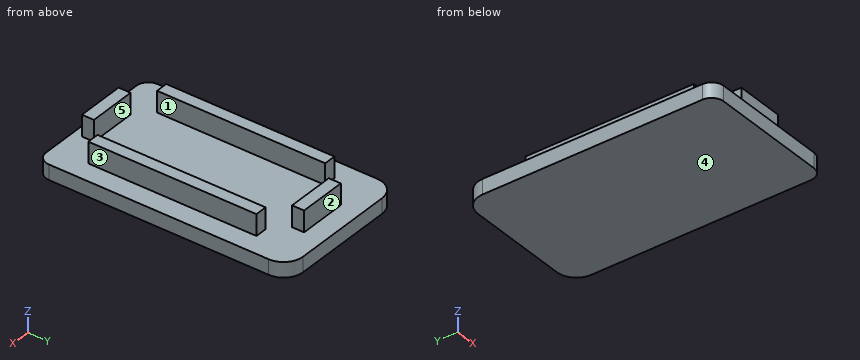
Autodesk Inventor part; units mm, degrees
ref_plane "YZ Plane" through (0, 0, 0) normal (1, 0, 0) x (0, 1, 0)
ref_plane "XZ Plane" through (0, 0, 0) normal (0, 1, 0) x (-1, 0, 0)
ref_plane "XY Plane" through (0, 0, 0) normal (0, 0, 1) x (1, 0, 0)
sketch "Boceto1" plane through (0, 0, 0) normal (0, 0, 1) x (1, 0, 0)
  line L0 (20, -40) -> (-20, -40)
  line L1 (-20, -40) -> (-20, 40)
  line L2 (-20, 40) -> (20, 40)
  line L3 (20, 40) -> (20, -40)
  line L4 (20, -40) -> (-20, 40) construction
  line L5 (-20, -40) -> (20, 40) construction
  line L6 (23.7, -43.7) -> (-23.7, -43.7)
  line L7 (-23.7, -43.7) -> (-23.7, 43.7)
  line L8 (-23.7, 43.7) -> (23.7, 43.7)
  line L9 (23.7, 43.7) -> (23.7, -43.7)
  line L10 (-23.7, -40) -> (23.7, -40)
  point P0 (0, 0)
  dimension "d0" = 40
  dimension "d1" = 80
  dimension "d2" = 3.7
  dimension "d20" = 3.7
extrude "Extrusión1" add sketch "Boceto1" along normal blind 5 contours L0 L1 L2 L3 | L3 L2 L1 L10 L7 L8 L9
sketch "Boceto2" plane through (0, 0, 5) normal (0, 0, 1) x (1, 0, 0)
  line L0 (17.5, -37.5) -> (-17.5, -37.5)
  line L1 (-17.5, -37.5) -> (-17.5, 37.5)
  line L2 (-17.5, 37.5) -> (17.5, 37.5)
  line L3 (17.5, 37.5) -> (17.5, -37.5)
  line L4 (17.5, -37.5) -> (-17.5, 37.5) construction
  line L5 (-17.5, -37.5) -> (17.5, 37.5) construction
  line L6 (17, 37) -> (-17, 37)
  line L7 (-17, 37) -> (-17, -37)
  line L8 (-17, -37) -> (17, -37)
  line L9 (17, -37) -> (17, 37)
  line L10 (-13, 33) -> (13, 33)
  line L11 (13, 33) -> (13, -33)
  line L12 (13, -33) -> (-13, -33)
  line L13 (-13, -33) -> (-13, 33)
  line L14 (8, 33) -> (8, 37)
  line L15 (-8, 33) -> (-8, 37)
  line L16 (13, 28) -> (17, 28)
  line L17 (13, -28) -> (17, -28)
  line L18 (-13, -28) -> (-17, -28)
  line L19 (-8, -33) -> (-8, -37)
  line L20 (8, -33) -> (8, -37)
  line L21 (-17, 28) -> (-13, 28)
  point P0 (0, 0)
  dimension "d5" = 35
  dimension "d6" = 75
  dimension "d7" = 0.5
  dimension "d8" = 4
  dimension "d9" = 5
  dimension "d10" = 5
  dimension "d11" = 5
  dimension "d12" = 5
  dimension "d13" = 5
  dimension "d14" = 5
  dimension "d15" = 5
  dimension "d16" = 5
extrude "Extrusión2" add sketch "Boceto2" along normal blind 7 contours L14 L10 L15 L6 | L9 L17 L11 L16 | L21 L13 L18 L7 | L8 L19 L12 L20
fillet "Empalme1" radius 6.5 2 edges at (23.7, 43.7, 2.5) (-23.7, 43.7, 2.5)
fillet "Empalme2" radius 4 2 edges at (-23.7, -40, 2.5) (23.7, -40, 2.5)
properties part number "Tapacanto delantero"
Design review of the part built by this model. Coordinates are the model's own, in mm. Face numbers are marked on the shaded views. A direction names the side the tool comes from. Give positions to 0.01 mm unless a question says otherwise; leave off trailing zeros. Loops run counter-clockwise (first coordinate to the right, second up) from the corner with the lowest first, then second, coordinate; pieces in that order, holes last. Notation, with made-up numbers: M 8.25,66 L 41.25,66 A30 cw 41.25,99 Z; hole C 67.25,27 d8. An arc over 180 degrees is marked long. Return JSON: item names as keys, results as strings. Group by question number.
Item 1: Mouldability with a two-part tool opening along X and no side actions: class the marked faces 1, 2 and 3 as released by +X, released by -X, zero draft, split by the parting line, or undercut.
Item 2: We need section D-D (y = 11). Give the boundary of the cut face in (x, z).
Item 3: Insertion check: pin 1 Ø4 at (y, z) = (23.5, 9) entering from +X; pin 2 Ø5.5 at (x, z) = (2.5, 8) entering from -Y; pin 3 Ø3.5 at (x, z) = (-1, 7.5) entering from +Y. Each pin has a flat end and moves straight along its axis. Give the tip position at first contact, or say it passes through.
Item 4: We need section C-C (x = 5). Give the boundary of the cut face in (y, z), and give its area (4 significant figures).
Item 5: Tool access review of the marked faces 4 and 5: name each direction out of +Z, -Z, +X, -X, +Y, -Y from which nothing blocks a thin tool from reaching the whole face with its end or side.
Item 6: For probe 1 along X at (y, z) = (-19, 10.5); probe 2 along Y at (x, z) = (1.5, 8.5); probe 3 along Z at (x, y) = (3, 15), list the stretches that pass through material, from the lowest coordinate up.
Item 7: We need section A-A (z = 9.5). Give the boundary of the cut face in (x, y).
Item 8: We need section B-B (y = -34). Give the boundary of the cut face in (x, z).
Output:
{
 "1": {"face 1": "undercut", "face 2": "zero draft", "face 3": "released by +X"},
 "2": {"outline": "M -23.7,0 L 23.7,0 L 23.7,5 L 17,5 L 17,12 L 13,12 L 13,5 L -13,5 L -13,12 L -17,12 L -17,5 L -23.7,5 Z"},
 "3": {"pin 1": "stops at x = 17", "pin 2": "stops at y = -37", "pin 3": "stops at y = 37"},
 "4": {"outline": "M -40,0 L 43.7,0 L 43.7,5 L 37,5 L 37,12 L 33,12 L 33,5 L -33,5 L -33,12 L -37,12 L -37,5 L -40,5 Z", "area": "474.5 mm^2"},
 "5": {"face 4": "-Z, +X, -X, +Y, -Y", "face 5": "+Z, +X, -X"},
 "6": {"probe 1": "x = -17 to -13, 13 to 17", "probe 2": "y = -37 to -33, 33 to 37", "probe 3": "z = 0 to 5"},
 "7": {"outline": "M -17,-28 L -13,-28 L -13,28 L -17,28 Z; M -8,-37 L 8,-37 L 8,-33 L -8,-33 Z; M -8,33 L 8,33 L 8,37 L -8,37 Z; M 13,-28 L 17,-28 L 17,28 L 13,28 Z"},
 "8": {"outline": "M -23.7,0 L 23.7,0 L 23.7,5 L 8,5 L 8,12 L -8,12 L -8,5 L -23.7,5 Z"}
}
